```python
from build123d import *

# Parameters (mm, degrees)
SKETCH1_W           = 30
SKETCH1_H           = 30
BOSS_EXTRUDE1_DEPTH = 6
CHAMFER1_SIZE       = 20


with BuildPart() as part:
    # Sketch1 → Boss-Extrude1 (new body)
    with BuildSketch(Plane(origin=(0, 0, 0), x_dir=(1, 0, 0), z_dir=(0, 1, 0))):
        Rectangle(SKETCH1_W, SKETCH1_H)
    extrude(amount=BOSS_EXTRUDE1_DEPTH)

    # Chamfer1
    chamfer1_edges = [part.edges().sort_by_distance(p)[0] for p in [
        (-15, 3, -15),
    ]]
    chamfer(chamfer1_edges, length=CHAMFER1_SIZE)


solid = part.part
```
Part model, mm, in its own coordinate system. Round coordinates to 2 decimals unless told otherwise and drop trailing zeros. Loops run counter-clockwise (first coordinate to the right, second up) from the corner with the lowest first, then second, coordinate; pieces in that order, holes last. Notation, with made-up numbers: (-17.75, -18.5) -> (21.25, -18.5) arc R22 ccw to (21.25, 19.5) -> close; hole circle Ø3 at (30.5, -11.75). An arc over 180 degrees is marked (long way). Use CSV: the item, a comma, the result in double quotes. Start each with the question number.
1) Drop a flat-ended pin along its axis: P1, Ø10, axis at x = 5.5, z = -3, coming from the -Y side. Give the stop position or say it passes through.
2) Cut at A-A, the plane z = -8.75. Write the cut outline in (x, y), plus the area to 3 significant figures.
3) Cut at C-C, the plane y = 0.5. Write the cut outline in (x, z), plus the area to 3 significant figures.
4) Cut at B-B, the plane x = -8. Write the cut outline in (y, z).
5) Wall check: L1, parallel to X at y = 5.5, z = -13; L2, parallel to Z at x = 3.75, y = 4.75; L3, parallel to X at y = 2.5, z = -10.5. Give the ranges that are in metal, low to high. Write a range as [from, to].
Determined:
1,P1,"stops at y = 0"
2,outline,"(-1.25, 0) -> (15, 0) -> (15, 6) -> (-1.25, 6) -> close"
2,area,"97.5 mm2"
3,outline,"(-15, 5) -> (5, -15) -> (15, -15) -> (15, 15) -> (-15, 15) -> close"
3,area,"700 mm2"
4,outline,"(0, -2) -> (6, -2) -> (6, 15) -> (0, 15) -> close"
5,L1,"x = [3, 15]"
5,L2,"z = [-13.75, 15]"
5,L3,"x = [0.5, 15]"
